Autodesk Inventor part; units mm, degrees
ref_plane "YZ Plane" through (0, 0, 0) normal (1, 0, 0) x (0, 1, 0)
ref_plane "XZ Plane" through (0, 0, 0) normal (0, 1, 0) x (-1, 0, 0)
ref_plane "XY Plane" through (0, 0, 0) normal (0, 0, 1) x (1, 0, 0)
sketch "Sketch1" plane through (0, 0, 0) normal (0, 0, 1) x (1, 0, 0)
  line L0 (0, 0) -> (23.0859, 0)
  line L1 (0, 17.5) -> (10, 17.5)
  line L2 (10, 17.5) -> (10, 26)
  line L3 (10, 26) -> (25, 26)
  line L4 (0, 22.5) -> (0, 17.5)
  line L5 (2, 22.5) -> (2, 40)
  line L6 (2, 40) -> (8, 40)
  line L7 (8, 40) -> (8, 30)
  line L8 (8, 30) -> (25, 30)
  line L9 (25, 30) -> (25, 26)
  line L10 (0, 22.5) -> (2, 22.5)
  dimension "d0" = 35
  dimension "d1" = 52
  dimension "d2" = 15
  dimension "d3" = 6
  dimension "d4" = 80
  dimension "d5" = 60
  dimension "d6" = 45
  dimension "d7" = 25
  dimension "d8" = 8
revolve "Revolution1" add sketch "Sketch1" angle 360 about axis through (0, 0, 0) along (1, 0, 0)
fillet "Fillet1" radius 2 3 edges at (2, -22.5, 0) (8, -30, 0) (10, -26, 0)
chamfer "Chamfer1" distance 1 angle 45 2 edges at (25, -30, 0) (2, -40, 0)
properties part number "CoverOutput"
Input: part model. Units: mm. Frame: model coordinates. A direction names the side the tool comes from. Round coordinates to 2 decimals unless told otherwise and drop trailing zeros. Order: outer loops, then holes, each group sorted by start corner. A loop starts at its lowest first (then second) coordinate and runs counter-clockwise, first axis right, second up.
1. Cut plane D-D, the plane x = 9. Output: boundary loops of the cut face in (y, z), then the cut area to 3 significant figures.
The answers:
outline: circle Ø60.54 at (0, 0); hole circle Ø35 at (0, 0)
area: 1,920 mm2
2. Set-up query: faces 4 (the face through (5.07, -13.887, -10.648)), 5 (the face through (8, -18, 27)), 6 (the face through (2, 17, 18)). Return all of +Z, -Z, +X, -X, +Y, -Y with unobstructed straight access to the full face (end or side cutting, diameter ignored); none if empty.
The answers:
face 4: +X, -X
face 5: +X
face 6: -X
3. Mould query, pull axis Z, two halves, no side actions, for faces 1 (the face through (17.1, -29.97, 1.32)), 2 (the face through (25, -11, 24)), 3 (the face through (10, 2, -18)). Classes: released by +Z, released by -Z, zero draft, split by the parting line, or undercut.
The answers:
face 1: split by the parting line
face 2: zero draft
face 3: undercut
4. Cut plane C-C, the plane x = 21. Output: boundary loops of the cut face in (y, z).
The answers:
outline: circle Ø60 at (0, 0); hole circle Ø52 at (0, 0)
5. Material intervals for line 1 (Z direction, x = 20, y = 0); line 2 (X direction, y = -28.5, z = -3); line 3 (Y direction, x = 15.25, z = 2.5), sorted ascending.
The answers:
line 1: z = -30 to -26, 26 to 30
line 2: x = 2 to 25
line 3: y = -29.9 to -25.88, 25.88 to 29.9
6. Pin query (flat end, axial travel): P1, Ø5, axis at x = 22, y = -9, coming from the +Z side; P2, Ø12, axis at x = 9, y = 14, coming from the -Z side; P3, Ø1.5, axis at x = 10, z = 4, coming from the +Y side. Return the tip coordinate at first contact, or that it passes through.
The answers:
P1: stops at z = 29.29
P2: stops at z = -39.17
P3: stops at y = 29.89
